Read the model definition and answer for the solid it produces. Units are mm, in the model's axes. A direction names the side the tool comes from. Coordinates: 2 decimals unless noted, no trailing zeros. Write each loop counter-clockwise with the first axis right and the second up, starting at its lowest first coordinate (ties: lowest second). Pieces come first, ordered by that corner, then holes.
(1) Find the intervals of material crossed by probe 1 along Y at (x, z) = (115, -24.5); probe 2 along X at (y, z) = (235, -32); probe 3 along Y at (x, z) = (-30, -32), in increasing order.
(2) Given pin 1 (5 mm diameter, centred on y = 199, z = -25, fed in from +X); pin 2 (16 mm diameter, centred on x = 115, y = 105, fed in from +Z); pin 3 (9 mm diameter, centred on x = 155, y = 235, fed in from -Z); pin 4 (11.5 mm diameter, centred on y = 260, z = -10, fed in from +X), each flat-ended and moving along its own axis, determine where each tip first touches the part or whether it passes through.
(3) Which of the six approach directions +Z, -Z, +X, -X, +Y, -Y give full straight-line access (tool end or side, diameter ignored) to faces 1 (the flat face through (152, 260, -10)), 2 (the flat face through (56, 225, -20)), 3 (the flat face through (94, 132.5, -30)), 4 (the flat face through (-2, 340, -20))?
(4) Section B-B on y = 170 is taken. Write down the section's boundary in (x, z), then the cut area to 3 significant figures.
(5) Section C-C on z = -25 is taken. State how many separate pieces and enclosed holes the cut face has, then the cut area to 3 significant figures.
(6) The mould has two halves that part along Z. Classify faces 5 (the cylindrical face through (159, 108, -30)), 6 (the flat face through (-76, 172, 0)), 7 (the flat face through (152, 80, -10)): +Z half, -Z half, draft (parallel to the pull), parting line (faces both ways), or undercut.
(7) Section D-D on y = 235 is taken. Write down the section's boundary in (x, z), then the cut area to 3 significant figures.
(8) Section A-A on x = 115 is taken. Write down the section's boundary in (y, z), then the cut area to 3 significant figures.
from build123d import *

# Parameters (mm, degrees)
SKETCH2_W               = 340
SKETCH2_H               = 340
BOSS_EXTRUDE1_DEPTH     = 40
CUT_EXTRUDE1_DEPTH      = 20
CUT_EXTRUDE2_DEPTH      = 100
CUT_EXTRUDE2_DEPTH_BACK = 199
SKETCH5_R               = 5
CUT_EXTRUDE4_DEPTH      = 363
CUT_EXTRUDE4_DEPTH_BACK = 260
SKETCH6_R               = 5
CUT_EXTRUDE5_DEPTH      = 18
FILLET1_R               = 3


with BuildPart() as part:
    # Sketch2 → Boss-Extrude1 (new body)
    with BuildSketch(Plane.XY):
        with Locations((0, 170)):
            Rectangle(SKETCH2_W, SKETCH2_H)
    extrude(amount=-BOSS_EXTRUDE1_DEPTH)

    # Sketch3 → Cut-Extrude1 (cut)
    with BuildSketch(Plane.XY):
        with BuildLine():
            ThreePointArc((20, 207.5), (-17.5, 170), (20, 132.5))
            Line((20, 132.5), (170, 132.5))
            Line((170, 132.5), (170, 89))
            Line((170, 89), (20, 89))
            ThreePointArc((20, 89), (-61, 170), (20, 251))
            Line((20, 251), (170, 251))
            Line((170, 251), (170, 207.5))
            Line((170, 207.5), (20, 207.5))
        make_face()
    extrude(amount=-CUT_EXTRUDE1_DEPTH, mode=Mode.SUBTRACT)

    # Sketch4 → Cut-Extrude2 (cut, two sides)
    with BuildSketch(Plane.XY) as cut_extrude2_sk:
        with BuildLine():
            Line((170, 132.5), (170, 207.5))
            Line((170, 207.5), (20, 207.5))
            ThreePointArc((20, 207.5), (-17.5, 170), (20, 132.5))
            Line((20, 132.5), (170, 132.5))
        make_face()
    extrude(amount=CUT_EXTRUDE2_DEPTH, mode=Mode.SUBTRACT)
    extrude(cut_extrude2_sk.sketch, amount=-CUT_EXTRUDE2_DEPTH_BACK, mode=Mode.SUBTRACT)

    # Sketch5 → Cut-Extrude4 (cut, two sides)
    with BuildSketch(Plane.XY) as cut_extrude4_sk:
        with Locations(Location((20, 235, 0), (0, 0, 180))):
            Circle(SKETCH5_R)
        with Locations(Location((20, 105, 0), (0, 0, 180))):
            Circle(SKETCH5_R)
        with Locations(Location((75, 235, 0), (0, 0, 180))):
            Circle(SKETCH5_R)
        with Locations(Location((75, 105, 0), (0, 0, 180))):
            Circle(SKETCH5_R)
        with Locations(Location((115, 235, 0), (0, 0, 180))):
            Circle(SKETCH5_R)
        with Locations(Location((155, 235, 0), (0, 0, 180))):
            Circle(SKETCH5_R)
        with Locations(Location((115, 105, 0), (0, 0, 180))):
            Circle(SKETCH5_R)
        with Locations(Location((155, 105, 0), (0, 0, 180))):
            Circle(SKETCH5_R)
        with Locations(Location((-25.961940777, 215.961940777, 0), (0, 0, 180))):
            Circle(SKETCH5_R)
        with Locations(Location((-45, 170, 0), (0, 0, 180))):
            Circle(SKETCH5_R)
        with Locations(Location((-25.961940777, 124.038059223, 0), (0, 0, 180))):
            Circle(SKETCH5_R)
    extrude(amount=CUT_EXTRUDE4_DEPTH, mode=Mode.SUBTRACT)
    extrude(cut_extrude4_sk.sketch, amount=-CUT_EXTRUDE4_DEPTH_BACK, mode=Mode.SUBTRACT)

    # Sketch6 → Cut-Extrude5 (cut)
    with BuildSketch(Plane(origin=(170, 0, 0), x_dir=(0, 0, -1), z_dir=(1, 0, 0))):
        with Locations(Location((10, 80, 0), (0, 0, 90))):
            Circle(SKETCH6_R)
        with Locations(Location((10, 310, 0), (0, 0, 90))):
            Circle(SKETCH6_R)
        with Locations(Location((10, 260, 0), (0, 0, 90))):
            Circle(SKETCH6_R)
        with Locations(Location((10, 30, 0), (0, 0, 90))):
            Circle(SKETCH6_R)
    extrude(amount=-CUT_EXTRUDE5_DEPTH, mode=Mode.SUBTRACT)

    # Fillet1
    fillet1_edges = [part.edges().sort_by_distance(p)[0] for p in [
        (0, 340, -40),
        (-170, 170, -40),
        (0, 340, 0),
        (0, 0, 0),
        (-170, 170, 0),
        (0, 0, -40),
    ]]
    fillet(fillet1_edges, radius=FILLET1_R)


solid = part.part
Response:
1. probe 1: y = 0 to 100, 110 to 132.5, 207.5 to 230, 240 to 340
1. probe 2: x = -170 to 15, 25 to 70, 80 to 110, 120 to 150, 160 to 170
1. probe 3: y = 0 to 121.09, 126.99 to 213.01, 218.91 to 340
2. pin 1: stops at x = -0.35
2. pin 2: stops at z = -20
2. pin 3: passes through
2. pin 4: stops at x = 170
3. face 1: +X
3. face 2: +Z, +X
3. face 3: +Z, -Z, +X
3. face 4: +Z, -Z, +X, -X, +Y
4. outline: (-170, -37) arc R3 ccw to (-167, -40) - (-50, -40) - (-50, -20) - (-61, -20) - (-61, 0) - (-167, 0) arc R3 ccw to (-170, -3) - close; (-40, -40) - (-17.5, -40) - (-17.5, -20) - (-40, -20) - close
4. area: 5,030 mm2
5. separate pieces: 1
5. enclosed holes: 11
5. area: 101,000 mm2
6. face 5: draft
6. face 6: +Z half
6. face 7: undercut
7. outline: (-170, -37) arc R3 ccw to (-167, -40) - (15, -40) - (15, -20) - (-28.33, -20) - (-28.33, 0) - (-167, 0) arc R3 ccw to (-170, -3) - close; (25, -40) - (70, -40) - (70, -20) - (25, -20) - close; (80, -40) - (110, -40) - (110, -20) - (80, -20) - close; (120, -40) - (150, -40) - (150, -20) - (120, -20) - close; (160, -40) - (170, -40) - (170, -20) - (160, -20) - close
7. area: 8,830 mm2
8. outline: (0, -37) arc R3 ccw to (3, -40) - (100, -40) - (100, -20) - (89, -20) - (89, 0) - (3, 0) arc R3 ccw to (0, -3) - close; (110, -40) - (132.5, -40) - (132.5, -20) - (110, -20) - close; (207.5, -40) - (230, -40) - (230, -20) - (207.5, -20) - close; (240, -40) - (337, -40) arc R3 ccw to (340, -37) - (340, -3) arc R3 ccw to (337, 0) - (251, 0) - (251, -20) - (240, -20) - close
8. area: 8,450 mm2
